Check sheet for the modelled part. Datum: model origin and axes. Units: mm. A direction names the side the tool comes from. Give positions to 0.01 mm unless a question says otherwise; leave off trailing zeros. Loops run counter-clockwise (first coordinate to the right, second up) from the corner with the lowest first, then second, coordinate; pieces in that order, holes last. Notation, with made-up numbers: (62.5, -12) - (92.5, -12) arc R22 cw to (92.5, 27) - close; hole circle Ø4 at (3.5, -21.5). An arc over 180 degrees is marked (long way). Answer in a Markdown table with one row per item. Add a question column.
(1) Sectioned sample at B-B on z = 26. Enter the section's corners in (x, y).
(2) Go/stop test with flat-tipped pins: P1, Ø12, axis at x = -109.5, y = -160.5, coming from the +Z side; P2, Ø3, axis at x = -70.5, z = 6.5, coming from the +Y side; P3, Ø5, axis at x = -287, z = 12, coming from the +Y side. Record where each tip stops, or that it passes through.
(3) Sectioned sample at D-D on x = -239. Enter the section's corners in (y, z), then the cut area to 3 significant figures.
(4) Sectioned sample at C-C on y = -44.5. Enter the section's corners in (x, z).
(5) Set-up check for faces 4 (the face through (-148, -101, 0)), 5 (the face through (-285, -2.4, 10)): record each of +Z, -Z, +X, -X, +Y, -Y from which the full face is reachable in a straight line by a thin tool's end or side.
(6) Draft check along X on faces 1 (the face through (-300, -79, 20)), 2 (the face through (-20, -107, 27)), 3 (the face through (0, -79, 20)). Enter one of: released by +X, released by -X, zero draft, split by the parting line, or undercut.
(7) Sectioned sample at A-A on x = -130. Enter the section's corners in (y, z).
(8) Thickness scan on L1, parallel to Z at x = -209.5, y = -118.5; L2, parallel to Z at x = -71.5, y = -89.5; L3, parallel to Y at x = -80.5, z = 40.5. Record the ranges inside material, lowest first.
from build123d import *

# Parameters (mm, degrees)
F1_DEPTH = 300
F3_W     = 197
F3_H     = 148
F4_DEPTH = 5
F6_DEPTH = 2.4


with BuildPart() as f1:
    # F0 (on Right) → F1 (new body)
    with BuildSketch(Plane.YZ):
        Polygon((-200, 10), (-200, 0), (0, 0), (0, 50), (-10, 50), align=None)
    extrude(amount=-F1_DEPTH)

    # F3 (on offset) → F4 (cut)
    with BuildSketch(Plane(origin=(0, -10.5039787798, 49.8938992042), x_dir=(1, 0, 0), z_dir=(0, -0.206010481, 0.978549785))):
        with Locations((-118.5, -98.4849737974)):
            Rectangle(F3_W, F3_H)
    extrude(amount=-F4_DEPTH, mode=Mode.SUBTRACT)

    # F5 (on face) → F6 (cut)
    with BuildSketch(Plane(origin=(0, 0, 0), x_dir=(-1, 0, 0), z_dir=(0, 1, 0))):
        with BuildLine():
            Line((277, 5), (293, 5))
            ThreePointArc((293, 5), (294.4142135624, 5.5857864376), (295, 7))
            Line((295, 7), (295, 13))
            ThreePointArc((295, 13), (294.4142135624, 14.4142135624), (293, 15))
            Line((293, 15), (277, 15))
            ThreePointArc((277, 15), (275.5857864376, 14.4142135624), (275, 13))
            Line((275, 13), (275, 7))
            ThreePointArc((275, 7), (275.5857864376, 5.5857864376), (277, 5))
        make_face()
    extrude(amount=-F6_DEPTH, mode=Mode.SUBTRACT)


solid = f1.part
Reply:
| question | item | result |
|---|---|---|
| 1 | outline | (-300, -124) - (-217, -124) - (-217, -99.73) - (-20, -99.73) - (-20, -124) - (0, -124) - (0, 0) - (-300, 0) - close |
| 2 | P1 | z = 14.47 |
| 2 | P2 | y = 0 |
| 2 | P3 | y = -2.4 |
| 3 | outline | (-200, 0) - (0, 0) - (0, 50) - (-10, 50) - (-200, 10) - close |
| 3 | area | 6,200 mm^2 |
| 4 | outline | (-300, 0) - (0, 0) - (0, 42.74) - (-20, 42.74) - (-20, 37.63) - (-217, 37.63) - (-217, 42.74) - (-300, 42.74) - close |
| 5 | face 4 | -Z, +X, -X, +Y, -Y |
| 5 | face 5 | +Y |
| 6 | face 1 | released by -X |
| 6 | face 2 | undercut |
| 6 | face 3 | released by +X |
| 7 | outline | (-200, 0) - (0, 0) - (0, 50) - (-10, 50) - (-34.46, 44.85) - (-33.43, 39.96) - (-178.26, 9.47) - (-179.29, 14.36) - (-200, 10) - close |
| 8 | L1 | 0 to 22.05 |
| 8 | L2 | 0 to 28.15 |
| 8 | L3 | -33.55 to 0 |
